Check sheet for the modelled part. Datum: model origin and axes. Units: mm. Face numbers are marked on the shaded views. A direction names the side the tool comes from. Give positions to 0.01 mm unless a question says otherwise; leave off trailing zeros. Order: outer loops, then holes, each group sorted by start corner. A loop starts at its lowest first (then second) coordinate and runs counter-clockwise, first axis right, second up.
from build123d import *

# Parameters (mm, degrees)
SKETCH1_W           = 40
SKETCH1_H           = 40
BOSS_EXTRUDE1_DEPTH = 30
SKETCH2_R           = 15
CUT_EXTRUDE1_DEPTH  = 41
CUT_EXTRUDE2_DEPTH  = 2.5


with BuildPart() as part:
    # Sketch1 → Boss-Extrude1 (new body)
    with BuildSketch(Plane.XY):
        with Locations((-30, 25)):
            Rectangle(SKETCH1_W, SKETCH1_H)
    extrude(amount=BOSS_EXTRUDE1_DEPTH)

    # Sketch2 → Cut-Extrude1 (cut, through all)
    with BuildSketch(Plane.XZ.offset(-5)):
        with Locations((-30, 30)):
            Circle(SKETCH2_R)
    extrude(amount=-CUT_EXTRUDE1_DEPTH, mode=Mode.SUBTRACT)

    # Sketch3 → Cut-Extrude2 (cut)
    with BuildSketch(Plane(origin=(0, 45, 0), x_dir=(1, 0, 0), z_dir=(0, 1, 0))):
        with BuildLine():
            Line((-10, -30), (-15, -30))
            ThreePointArc((-15, -30), (-30, -15), (-45, -30))
            Line((-45, -30), (-50, -30))
            Line((-50, -30), (-50, -9.862457081))
            Line((-50, -9.862457081), (-10, -9.862457081))
            Line((-10, -9.862457081), (-10, -30))
        make_face()
    extrude(amount=-CUT_EXTRUDE2_DEPTH, mode=Mode.SUBTRACT)


solid = part.part
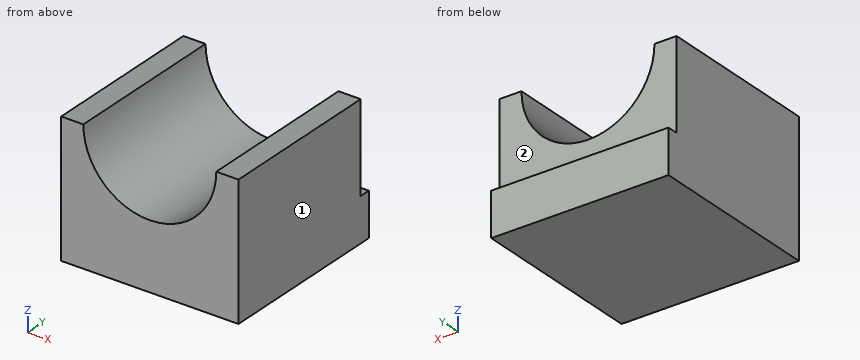
1) Section check C-C, the plane x = -23. Record the cut outline in (y, z).
Recorded:
outline: (5, 0) - (45, 0) - (45, 9.86) - (42.5, 9.86) - (42.5, 16.73) - (5, 16.73) - close
2) Section check A-A, the plane z = 25.5. Record the cut outline in (x, y).
Recorded:
outline: (-50, 5) - (-44.31, 5) - (-44.31, 42.5) - (-50, 42.5) - close; (-15.69, 5) - (-10, 5) - (-10, 42.5) - (-15.69, 42.5) - close
3) Depth check by flat-ended pin: pin 1 Ø1.5 at (x, z) = (-35.5, 15) entering from +Y; pin 2 Ø6 at (x, y) = (-25.5, 29) entering from +Z; pin 3 Ø0.8 at (x, y) = (-28, 43) entering from +Z. Enter the tip coordinate at first touch or a pass-through.
Recorded:
pin 1: stops at y = 42.5
pin 2: stops at z = 17.01
pin 3: stops at z = 9.86
4) Section check B-B, the plane y = 30. Record the cut outline in (x, z), then the cut area to 3 significant figures.
Recorded:
outline: (-50, 0) - (-10, 0) - (-10, 30) - (-15, 30) arc R15 cw to (-45, 30) - (-50, 30) - close
area: 847 mm2
5) Material ranges on L1, parallel to X at y = 7, z = 23.5; L2, parallel to X at y = 39, z = 28.5; L3, parallel to Y at x = -23.5, z = 10, recorded low to high.
Recorded:
L1: x = -50 to -43.52, -16.48 to -10
L2: x = -50 to -44.92, -15.08 to -10
L3: y = 5 to 42.5
6) Set-up check for the marked faces 1 and 2: record each of +Z, -Z, +X, -X, +Y, -Y from which the full face is reachable in a straight line by a thin tool's end or side.
Recorded:
face 1: +Z, -Z, +X, +Y, -Y
face 2: +Z, +X, -X, +Y
7) Section check D-D, the plane z = 22. Record the cut outline in (x, y).
Recorded:
outline: (-50, 5) - (-42.69, 5) - (-42.69, 42.5) - (-50, 42.5) - close; (-17.31, 5) - (-10, 5) - (-10, 42.5) - (-17.31, 42.5) - close
